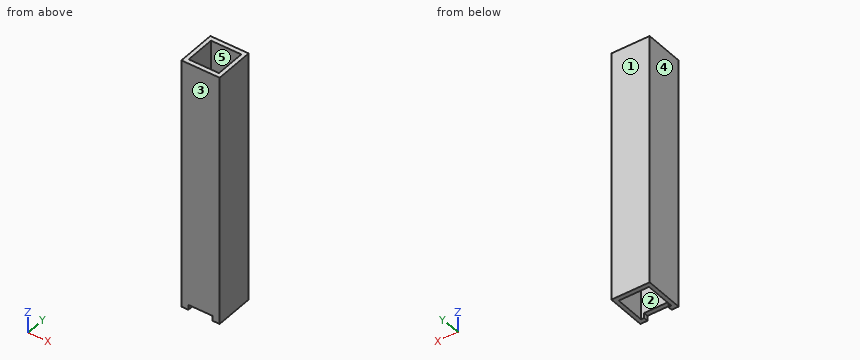
from build123d import *

# Parameters (mm, degrees)
SKETCH3_W           = 9.616935552
SKETCH3_H           = 9.912195066
SKETCH3_W_2         = 7.62
SKETCH3_H_2         = 7.62
BOSS_EXTRUDE2_DEPTH = 63.5
CUT_EXTRUDE1_DEPTH  = 1.27


with BuildPart() as part:
    # Sketch3 → Boss-Extrude2 (new body)
    with BuildSketch(Plane.XY):
        Rectangle(SKETCH3_W, SKETCH3_H)
        Rectangle(SKETCH3_W_2, SKETCH3_H_2, mode=Mode.SUBTRACT)
    extrude(amount=BOSS_EXTRUDE2_DEPTH)

    # Sketch6 → Cut-Extrude1 (cut)
    with BuildSketch(Plane(origin=(0, -3.81, 0), x_dir=(1, 0, 0), z_dir=(0, 1, 0))):
        Polygon((0, 0), (-3.048, 0), (-3.048, -1.27), (3.048, -1.27), (3.048, 0), align=None)
    extrude(amount=-CUT_EXTRUDE1_DEPTH, mode=Mode.SUBTRACT)


solid = part.part
Could you check a few things on this model? Use its own coordinates, in mm. Face numbers are marked on the shaded views. A direction names the side the tool comes from. Round coordinates to 2 decimals unless told otherwise and drop trailing zeros. Write each loop counter-clockwise with the first axis right and the second up, starting at its lowest first coordinate (ties: lowest second). Pieces come first, ordered by that corner, then holes. Notation, with made-up numbers: (-28.75, 39.25) -> (23.25, 39.25) arc R16 ccw to (23.25, 70.25) -> close; hole circle Ø6 at (-21.75, 28). An arc over 180 degrees is marked (long way). Use a Markdown table: item, result.
1. For pin 1 Ø0.6 at (x, y) = (0, -4.5) entering from -Z, with a flat end and sliding along its axis, tell me the tip position at first contact or that it passes through.
Answer key:
| item | result |
|---|---|
| pin 1 | stops at z = 1.27 |
2. We'd pull the mould along X, two halves only. Please class the marked faces 3, 4 and 5: +X half, -X half, draft (parallel to the pull), parting line (faces both ways), or undercut.
Answer key:
| item | result |
|---|---|
| face 3 | draft |
| face 4 | -X half |
| face 5 | undercut |
3. If we section it at C-C (x = -1.5): List the corners of the cut face in (y, z) for me.
Answer key:
| item | result |
|---|---|
| outline | (-4.96, 1.27) -> (-3.81, 1.27) -> (-3.81, 63.5) -> (-4.96, 63.5) -> close; (3.81, 0) -> (4.96, 0) -> (4.96, 63.5) -> (3.81, 63.5) -> close |
4. If we section it at B-B (z = 33): List the corners of the cut face in (x, y) for me, then the cut area to 3 significant figures.
Answer key:
| item | result |
|---|---|
| outline | (-4.81, -4.96) -> (4.81, -4.96) -> (4.81, 4.96) -> (-4.81, 4.96) -> close; hole (-3.81, -3.81) -> (3.81, -3.81) -> (3.81, 3.81) -> (-3.81, 3.81) -> close |
| area | 37.3 mm^2 |
5. If we section it at A-A (y = -2.5): List the corners of the cut face in (x, z) for me.
Answer key:
| item | result |
|---|---|
| outline | (-4.81, 0) -> (-3.81, 0) -> (-3.81, 63.5) -> (-4.81, 63.5) -> close; (3.81, 0) -> (4.81, 0) -> (4.81, 63.5) -> (3.81, 63.5) -> close |
6. Please list where these lines run through material, in increasing order: probe 1 along X at (y, z) = (-3.75, 43.5); probe 2 along Y at (x, z) = (1.5, 44.5).
Answer key:
| item | result |
|---|---|
| probe 1 | x = -4.81 to -3.81, 3.81 to 4.81 |
| probe 2 | y = -4.96 to -3.81, 3.81 to 4.96 |
7. Which directions (+Z, -Z, +X, -X, +Y, -Y) give clear straight access to the entire face, cutting with the end or side of a thin tool? Please do the marked faces 1 and 2.
Answer key:
| item | result |
|---|---|
| face 1 | +Z, -Z, +X, -X, +Y |
| face 2 | +Z, -Z |
